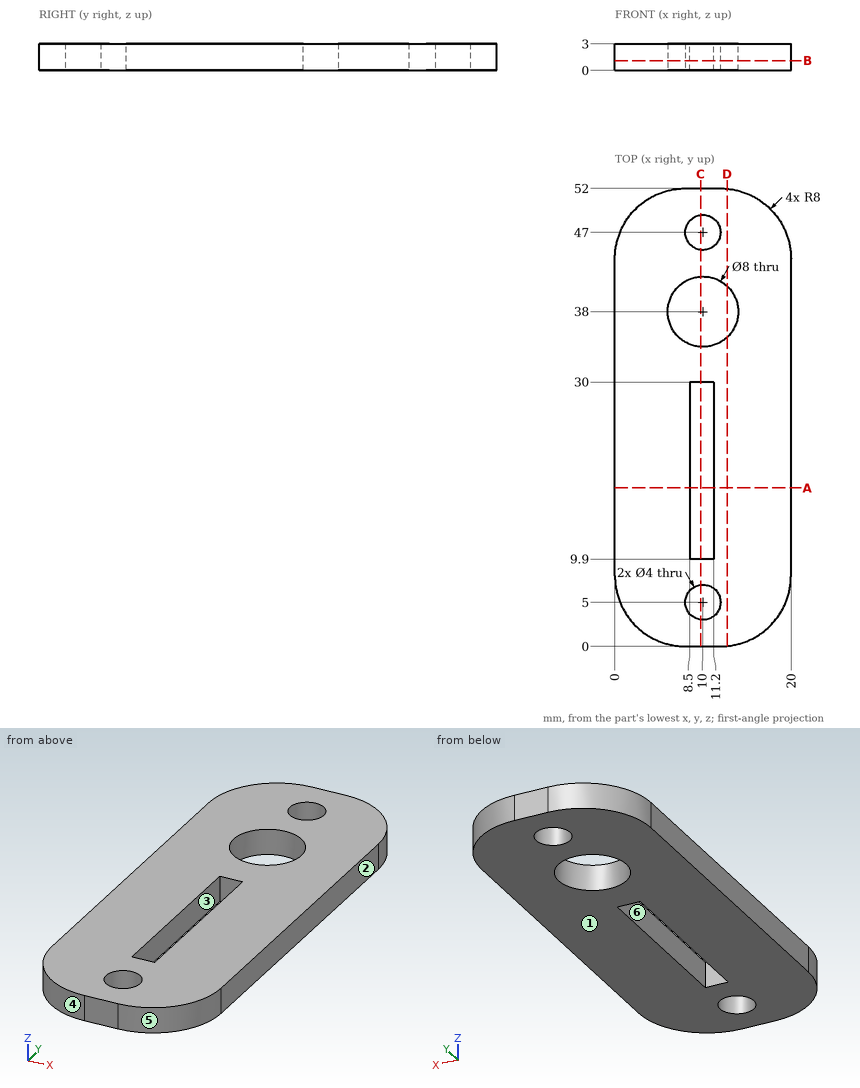
Answer from the drawing. Dimensions are ordinates in mm from the lowest x, y and z of the part. A direction names the side the tool comes from. Round coordinates to 2 decimals unless told otherwise and drop trailing zeros. Write each loop counter-clockwise with the first axis right and the second up, starting at its lowest first coordinate (ties: lowest second). Pieces come first, ordered by that corner, then holes. Notation, with made-up numbers: (-13, 18.25) -> (39, 18.25) arc R6 ccw to (39, 23.25) -> close; hole circle Ø11 at (78, 37). An arc over 180 degrees is marked (long way). Answer in a Markdown table with one row per item. Add a question column.
1) Determine the mould class of the marked faces 1, 2, 3 and 4 for opening direction X: pulls with the +X half, pulls with the -X half, needs draft (parallel to the pull), parting line crosses it, or undercut.
2) Consider line 1 (Y direction, x = 10, z = 0.7); line 2 (X direction, y = 38, z = 0.9); line 3 (X direction, y = 17, z = 2.05). Determine where each line is inside the solid, lowest interval first.
3) Which of the six approach directions +Z, -Z, +X, -X, +Y, -Y give full straight-line access (tool end or side, diameter ignored) to the marked faces 5 and 6?
4) Given P1, Ø4, axis at x = 17.5, y = 18, coming from the -Z side; P2, Ø1.5, axis at x = 15.5, z = 1.5, coming from the -Y side; P3, Ø1.5, axis at y = 46.5, z = 0.5, coming from the -X side, each flat-ended and moving along its own axis, determine where each tip first touches the part or whether it passes through.
5) Find section A-A, the plane y = 18. Determine the outline of the cut face in (x, z).
6) Find section C-C, the plane x = 9.75. Determine the outline of the cut face in (y, z).
7) Find section D-D, the plane x = 12.75. Determine the outline of the cut face in (y, z), and give its area (3 significant figures).
8) Find section B-B, the plane z = 1.1. Determine the outline of the cut face in (x, y).
Findings below:
| question | item | result |
|---|---|---|
| 1 | face 1 | needs draft |
| 1 | face 2 | pulls with the +X half |
| 1 | face 3 | undercut |
| 1 | face 4 | pulls with the -X half |
| 2 | line 1 | 0 to 3, 7 to 9.9, 30 to 34, 42 to 45, 49 to 52 |
| 2 | line 2 | 0 to 6, 14 to 20 |
| 2 | line 3 | 0 to 8.5, 11.2 to 20 |
| 3 | face 5 | +Z, -Z, +X, -Y |
| 3 | face 6 | +Z, -Z |
| 4 | P1 | z = 0 |
| 4 | P2 | y = 0.49 |
| 4 | P3 | x = 0.19 |
| 5 | outline | (0, 0) -> (8.5, 0) -> (8.5, 3) -> (0, 3) -> close; (11.2, 0) -> (20, 0) -> (20, 3) -> (11.2, 3) -> close |
| 6 | outline | (0, 0) -> (3.02, 0) -> (3.02, 3) -> (0, 3) -> close; (6.98, 0) -> (9.9, 0) -> (9.9, 3) -> (6.98, 3) -> close; (30, 0) -> (34.01, 0) -> (34.01, 3) -> (30, 3) -> close; (41.99, 0) -> (45.02, 0) -> (45.02, 3) -> (41.99, 3) -> close; (48.98, 0) -> (52, 0) -> (52, 3) -> (48.98, 3) -> close |
| 7 | outline | (0.04, 0) -> (35.1, 0) -> (35.1, 3) -> (0.04, 3) -> close; (40.9, 0) -> (51.96, 0) -> (51.96, 3) -> (40.9, 3) -> close |
| 7 | area | 138 mm² |
| 8 | outline | (0, 8) arc R8 ccw to (8, 0) -> (12, 0) arc R8 ccw to (20, 8) -> (20, 44) arc R8 ccw to (12, 52) -> (8, 52) arc R8 ccw to (0, 44) -> close; hole circle Ø8 at (10, 38); hole circle Ø4 at (10, 5); hole circle Ø4 at (10, 47); hole (8.5, 9.9) -> (11.2, 9.9) -> (11.2, 30) -> (8.5, 30) -> close |
